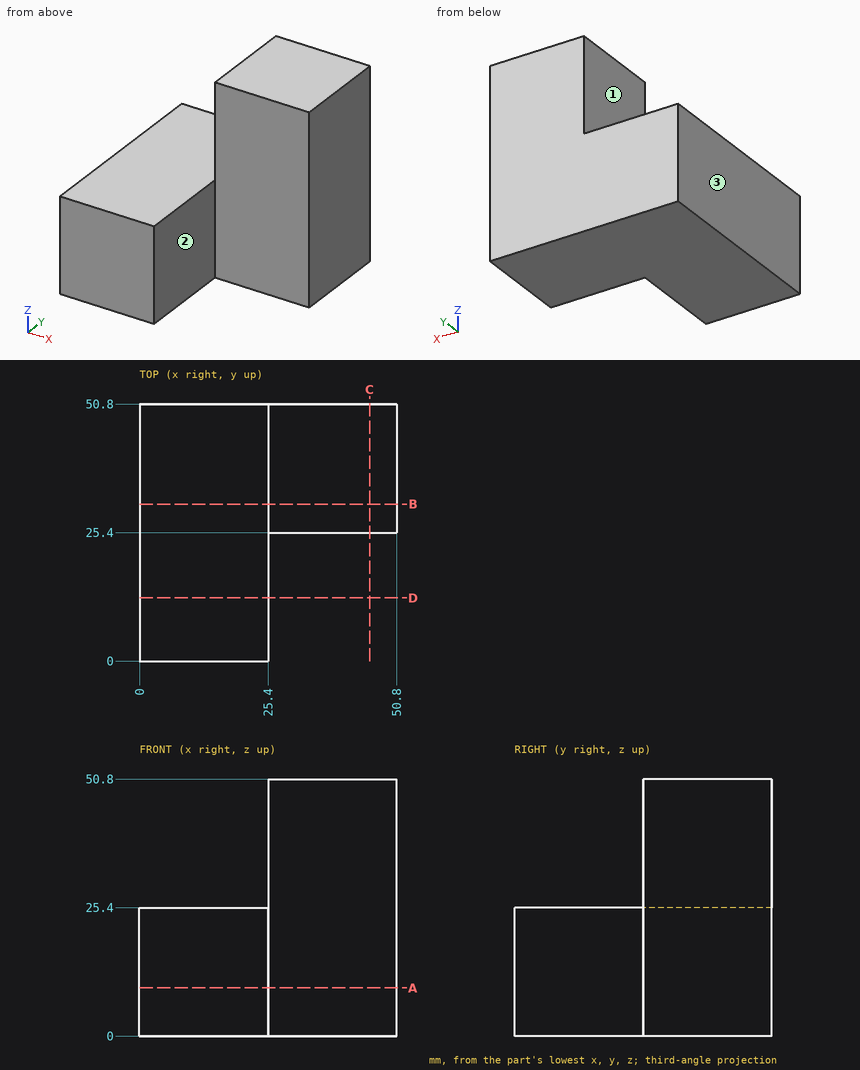
Source: three-view drawing plus pictorial views. Frame: mm from the lowest corner of the part. A direction names the side the tool comes from. Round coordinates to 2 decimals unless told otherwise and drop trailing zeros. Write each loop counter-clockwise with the first axis right and the second up, starting at its lowest first coordinate (ties: lowest second). Pieces come first, ordered by that corner, then holes. Notation, with made-up numbers: M 17,14.5 L 60,14.5 A30 ccw 60,36.5 Z; hole C 23,72 d5. An arc over 180 degrees is marked long. One line per item, written item: value. Start each with the question number.
Item 1: Set-up query: the marked faces 1, 2 and 3. Return all of +Z, -Z, +X, -X, +Y, -Y with unobstructed straight access to the full face (end or side cutting, diameter ignored); none if empty.
Item 2: Section query B-B (y = 31). Return the cut outline in (x, z), plus the area to 3 significant figures.
Item 3: Section query C-C (x = 45.5). Return the cut outline in (y, z), plus the area to 3 significant figures.
Item 4: Pin query (flat end, axial travel): pin 1 (5 mm diameter, centred on x = 42, z = 37.5, fed in from -Y); pin 2 (12.5 mm diameter, centred on x = 14, y = 29.5, fed in from +Z); pin 3 (20.5 mm diameter, centred on y = 35, z = 39.5, fed in from -X); pin 4 (6 mm diameter, centred on x = 32.5, y = 21, fed in from -Z). Return the tip coordinate at first contact, or that it passes through.
Item 5: Ray query, L1, parallel to X at y = 4.5, z = 10.5; L2, parallel to Y at x = 42.5, z = 36.5. Return the intervals inside material, ascending. Write a range as from..to.
Item 6: Section query A-A (z = 9.5). Return the cut outline in (x, y).
Item 7: Section query D-D (y = 12.5). Return the cut outline in (x, z).
Result set:
1. face 1: +Z, -X, +Y, -Y
1. face 2: +Z, -Z, +X, -Y
1. face 3: +Z, -Z, -X, +Y, -Y
2. outline: M 0,0 L 50.8,0 L 50.8,50.8 L 25.4,50.8 L 25.4,25.4 L 0,25.4 Z
2. area: 1,940 mm²
3. outline: M 25.4,0 L 50.8,0 L 50.8,50.8 L 25.4,50.8 Z
3. area: 1,290 mm²
4. pin 1: stops at y = 25.4
4. pin 2: stops at z = 25.4
4. pin 3: stops at x = 25.4
4. pin 4: passes through
5. L1: x = 0..25.4
5. L2: y = 25.4..50.8
6. outline: M 0,0 L 25.4,0 L 25.4,25.4 L 50.8,25.4 L 50.8,50.8 L 0,50.8 Z
7. outline: M 0,0 L 25.4,0 L 25.4,25.4 L 0,25.4 Z
